```python
from build123d import *

# Parameters (mm, degrees)
SKETCH_1_W          = 58
SKETCH_1_H          = 42
SKETCH_1_R          = 1.5
EXTRUDE_1_DEPTH     = 15
SKETCH_2_W          = 13.679310014
SKETCH_2_H          = 5.381736476
CUT_EXTRUDE_1_DEPTH = 12
SKETCH_3_W          = 17.182547944
SKETCH_3_H          = 10.048106392
CUT_EXTRUDE_2_DEPTH = 9
SKETCH_4_W          = 6.72992405
SKETCH_4_H          = 5.024053196
EXTRUDE_2_DEPTH     = 9


with BuildPart() as part:
    # 草图1 → 凸台-拉伸1 (new body)
    with BuildSketch(Plane(origin=(0, 0, 0), x_dir=(1, 0, 0), z_dir=(0, 1, 0))):
        Rectangle(SKETCH_1_W, SKETCH_1_H)
        with Locations(Location((-24.5, 17, 0), (0, 0, 270))):
            Circle(SKETCH_1_R, mode=Mode.SUBTRACT)
        with Locations(Location((-24.5, -17, 0), (0, 0, 90))):
            Circle(SKETCH_1_R, mode=Mode.SUBTRACT)
        with Locations(Location((24.5, -17, 0), (0, 0, 270))):
            Circle(SKETCH_1_R, mode=Mode.SUBTRACT)
        with Locations(Location((24.5, 17, 0), (0, 0, 90))):
            Circle(SKETCH_1_R, mode=Mode.SUBTRACT)
    extrude(amount=EXTRUDE_1_DEPTH)

    # 草图2 → 切除-拉伸1 (cut)
    with BuildSketch(Plane(origin=(0, 15, 0), x_dir=(1, 0, 0), z_dir=(0, 1, 0))):
        with Locations((0, 21)):
            Rectangle(SKETCH_2_W, SKETCH_2_H)
    extrude(amount=-CUT_EXTRUDE_1_DEPTH, mode=Mode.SUBTRACT)

    # 草图3 → 切除-拉伸2 (cut)
    with BuildSketch(Plane(origin=(0, 15, 0), x_dir=(1, 0, 0), z_dir=(0, 1, 0))):
        with Locations((0, -21)):
            Rectangle(SKETCH_3_W, SKETCH_3_H)
    extrude(amount=-CUT_EXTRUDE_2_DEPTH, mode=Mode.SUBTRACT)

    # 草图4 → 凸台-拉伸2 (add)
    with BuildSketch(Plane(origin=(0, 6, 0), x_dir=(1, 0, 0), z_dir=(0, 1, 0))):
        with Locations((0.325641486, -18.487973402)):
            Rectangle(SKETCH_4_W, SKETCH_4_H)
    extrude(amount=EXTRUDE_2_DEPTH)


solid = part.part
```
Work out the finished part from the listing and answer in its coordinate system (mm). A direction names the side the tool comes from. Coordinates: 2 decimals unless noted, no trailing zeros. Loops run counter-clockwise (first coordinate to the right, second up) from the corner with the lowest first, then second, coordinate; pieces in that order, holes last. Notation, with made-up numbers: (41.5, 44) - (63.5, 44) arc R17 ccw to (63.5, 63) - close; hole circle Ø2 at (18.5, 62.25). An arc over 180 degrees is marked (long way). Use a Markdown table: item, result.
Item 1: Given pin 1 Ø0.8 at (x, z) = (2.5, -20) entering from +Y; pin 2 Ø1.5 at (x, z) = (6, 19) entering from +Y; pin 3 Ø6 at (x, y) = (3.5, 11.5) entering from -Z, each flat-ended and moving along its own axis, determine where each tip first touches the part or whether it passes through.
Evaluation:
| item | result |
|---|---|
| pin 1 | stops at y = 3 |
| pin 2 | stops at y = 6 |
| pin 3 | stops at z = -18.31 |
Item 2: Find section C-C, the plane x = 24.5. Determine the outline of the cut face in (y, z).
Evaluation:
| item | result |
|---|---|
| outline | (0, -21) - (15, -21) - (15, -18.5) - (0, -18.5) - close; (0, -15.5) - (15, -15.5) - (15, 15.5) - (0, 15.5) - close; (0, 18.5) - (15, 18.5) - (15, 21) - (0, 21) - close |
Item 3: For faces 1 (the flat face through (8.591, 11, 19)), 2 (the flat face through (-6.84, 9, -20)), 3 (the flat face through (29, 7, 0)), determine the directions among +Z, -Z, +X, -X, +Y, -Y from which every point of the face is accessible in a straight line to the end or side of a thin tool.
Evaluation:
| item | result |
|---|---|
| face 1 | +Z, +Y |
| face 2 | -Z, +Y |
| face 3 | +Z, -Z, +X, +Y, -Y |
Item 4: The mould has two halves that part along X. Classify faces 4 (the flat face through (-6, 11, 15.976)), 5 (the flat face through (0, 7, 21)), 6 (the flat face through (0, 9, -18.309)), 7 (the flat face through (-29, 7, 0)): +X half, -X half, draft (parallel to the pull), parting line (faces both ways), or undercut.
Evaluation:
| item | result |
|---|---|
| face 4 | undercut |
| face 5 | draft |
| face 6 | undercut |
| face 7 | -X half |
Item 5: Find section D-D, the plane z = 17. Determine the outline of the cut face in (x, y).
Evaluation:
| item | result |
|---|---|
| outline | (-29, 0) - (-26, 0) - (-26, 15) - (-29, 15) - close; (-23, 0) - (23, 0) - (23, 15) - (8.59, 15) - (8.59, 6) - (3.69, 6) - (3.69, 15) - (-3.04, 15) - (-3.04, 6) - (-8.59, 6) - (-8.59, 15) - (-23, 15) - close; (26, 0) - (29, 0) - (29, 15) - (26, 15) - close |
Item 6: Consider probe 1 along X at (y, z) = (10.75, 17); probe 2 along X at (y, z) = (3.5, 17); probe 3 along X at (y, z) = (7.25, 17.5). Determine where each line is inside the solid, lowest interval first. Write a range as from..to.
Evaluation:
| item | result |
|---|---|
| probe 1 | x = -29..-26, -23..-8.59, -3.04..3.69, 8.59..23, 26..29 |
| probe 2 | x = -29..-26, -23..23, 26..29 |
| probe 3 | x = -29..-25.91, -23.09..-8.59, -3.04..3.69, 8.59..23.09, 25.91..29 |
Item 7: Find section B-B, the plane y = 4.75. Determine the outline of the cut face in (x, z).
Evaluation:
| item | result |
|---|---|
| outline | (-29, -21) - (-6.84, -21) - (-6.84, -18.31) - (6.84, -18.31) - (6.84, -21) - (29, -21) - (29, 21) - (-29, 21) - close; hole circle Ø3 at (-24.5, -17); hole circle Ø3 at (-24.5, 17); hole circle Ø3 at (24.5, -17); hole circle Ø3 at (24.5, 17) |
Item 8: Find section A-A, the plane z = -17. Determine the outline of the cut face in (x, y).
Evaluation:
| item | result |
|---|---|
| outline | (-29, 0) - (-26, 0) - (-26, 15) - (-29, 15) - close; (-23, 0) - (23, 0) - (23, 15) - (-23, 15) - close; (26, 0) - (29, 0) - (29, 15) - (26, 15) - close |
